```python
from build123d import *

# Parameters (mm, degrees)
F0_W      = 170
F0_H      = 145
F1_DEPTH  = 2
F2_R      = 2.45
F3_DEPTH  = 33
F4_W      = 10
F4_H      = 10
F5_DEPTH  = 20
F8_DEPTH  = 2
F9_W      = 8
F9_H      = 8
F10_DEPTH = 2


with BuildPart() as f1:
    # F0 (on Top) → F1 (new body)
    with BuildSketch(Plane.XY):
        with Locations((85, 72.5)):
            Rectangle(F0_W, F0_H)
    extrude(amount=F1_DEPTH)

    # F2 (on face) → F3 (join)
    with BuildSketch(Plane.XY.offset(2)):
        with Locations((22, 135.5)):
            Circle(F2_R)
        with Locations((22, 14.5)):
            Circle(F2_R)
        with Locations((143, 135.5)):
            Circle(F2_R)
        with Locations((143, 14.5)):
            Circle(F2_R)
    extrude(amount=F3_DEPTH)

    # F4 (on face) → F5 (join)
    with BuildSketch(Plane.XY.offset(2)):
        with Locations((85, 14.5)):
            Rectangle(F4_W, F4_H)
        with Locations((85, 135.5)):
            Rectangle(F4_W, F4_H)
        with Locations((22, 72.5)):
            Rectangle(F4_W, F4_H)
        with Locations((148, 72.5)):
            Rectangle(F4_W, F4_H)
    extrude(amount=F5_DEPTH)

    # F7 (on face) → F8 (join)
    with BuildSketch(Plane.XY.offset(2)):
        Polygon((85, 19.5), (27, 72.5), (27, 67.5), (22, 67.5), (80, 14.5), (80, 19.5), align=None)
        Polygon((143, 72.5), (85, 19.5), (90, 19.5), (90, 14.5), (148, 67.5), (143, 67.5), align=None)
        Polygon((90, 130.5), (85, 130.5), (143, 72.5), (143, 77.5), (148, 77.5), (90, 135.5), align=None)
        Polygon((27, 77.5), (27, 72.5), (85, 130.5), (80, 130.5), (80, 135.5), (22, 77.5), align=None)
    extrude(amount=F8_DEPTH)

    # F9 (on face) → F10 (join)
    with BuildSketch(Plane.XY.offset(2)):
        Polygon((31.1801801802, 68.6801801802), (81, 68.6801801802), (81, 76.6801801802), (31.1801801802, 76.6801801802), (27, 72.5), align=None)
        Polygon((81, 126.5), (81, 76.6801801802), (89, 76.6801801802), (89, 126.5), (85, 130.5), align=None)
        with Locations((85, 72.6801801802)):
            Rectangle(F9_W, F9_H)
        Polygon((143, 72.5), (138.8198198198, 68.6801801802), (139.1801801802, 68.6801801802), align=None)
        Polygon((89, 76.6801801802), (89, 68.6801801802), (138.8198198198, 68.6801801802), (143, 72.5), (138.8198198198, 76.6801801802), align=None)
        Polygon((81, 68.6801801802), (81, 23.1551724138), (85, 19.5), (89, 23.1551724138), (89, 68.6801801802), align=None)
    extrude(amount=F10_DEPTH)


solid = f1.part
```
CAD build for the part. Positions are in the model's coordinates, mm. A direction names the side the tool comes from. Give positions to 0.01 mm unless a question says otherwise; leave off trailing zeros. Loops run counter-clockwise (first coordinate to the right, second up) from the corner with the lowest first, then second, coordinate; pieces in that order, holes last. Notation, with made-up numbers: (-31, 20.5) - (27, 20.5) arc R19 cw to (27, 41.5) - close; hole circle Ø3 at (36, 74.5). An arc over 180 degrees is marked (long way). Put each result on its own line as item: value.
Q1. Tool access for faces 1 (the face through (145.263, 13.562, 18.269)), 2 (the face through (27, 72, 13)), 3 (the face through (17, 72, 12)), 4 (the face through (143, 15, 35)): list every direction of +Z, -Z, +X, -X, +Y, -Y with a clear straight run to the whole face (end or side of a thin tool).
Filled in:
face 1: +Z
face 2: +Z, +Y, -Y
face 3: +Z, -X, +Y, -Y
face 4: +Z, +X, -X, +Y, -Y
Q2. Slice it at A-A (y = 86.5). Give the cut face in (x, z).
Filled in:
outline: (0, 0) - (170, 0) - (170, 2) - (139, 2) - (139, 4) - (129, 4) - (129, 2) - (89, 2) - (89, 4) - (81, 4) - (81, 2) - (41, 2) - (41, 4) - (31, 4) - (31, 2) - (0, 2) - close
Q3. Probe line 1 along Z through (x, y) = (151, 130); line 2 along Y through (x, z) = (101, 3.5); line 3 along Z through (x, y) = (35, 70). List the from-to ranges inside material, lowest first.
Filled in:
line 1: z = 0 to 2
line 2: y = 24.55 to 34.12, 68.68 to 76.68, 114.5 to 124.5
line 3: z = 0 to 4
Q4. Mould opens along Y. For faces 5 (the face through (85, 9.5, 12)), 6 (the face through (20.056, 13.009, 18.269)), 7 (the face through (84, 74, 0)), 8 (the face through (143, 72, 13)) say: pulls with the +Y half, pulls with the -Y half, needs draft (parallel to the pull), parting line crosses it, or undercut.
Filled in:
face 5: pulls with the -Y half
face 6: undercut
face 7: needs draft
face 8: undercut
Q5. Flat gauge pins, fed straight in: pin 1 (10 mm diameter, centred on y = 31, z = 13, fed in from -X); pin 2 (11 mm diameter, centred on x = 84.5, z = 8.5, fed in from +Y); pin 3 (3 mm diameter, centred on y = 136, z = 13.5, fed in from -X); pin 4 (5 mm diameter, centred on x = 146.5, z = 14.5, fed in from -Y). Where does each tip first touch, or does it go through?
Filled in:
pin 1: passes through
pin 2: stops at y = 140.5
pin 3: stops at x = 19.55
pin 4: stops at y = 12.26
Q6. Slice it at C-C (z = 25.5). Give the cut face in (x, y), plus the area to 3 significant figures.
Filled in:
outline: circle Ø4.9 at (22, 14.5); circle Ø4.9 at (22, 135.5); circle Ø4.9 at (143, 14.5); circle Ø4.9 at (143, 135.5)
area: 75.4 mm²
Q7. Slice it at B-B (z = 16). Give the cut face in (x, y), plus the area to 3 significant figures.
Filled in:
outline: (17, 67.5) - (27, 67.5) - (27, 77.5) - (17, 77.5) - close; circle Ø4.9 at (22, 14.5); circle Ø4.9 at (22, 135.5); (80, 9.5) - (90, 9.5) - (90, 19.5) - (80, 19.5) - close; (80, 130.5) - (90, 130.5) - (90, 140.5) - (80, 140.5) - close; circle Ø4.9 at (143, 14.5); circle Ø4.9 at (143, 135.5); (143, 67.5) - (153, 67.5) - (153, 77.5) - (143, 77.5) - close
area: 475 mm²
Q8. Slice it at D-D (x = 71). Give the cut face in (y, z), plus the area to 3 significant figures.
Filled in:
outline: (0, 0) - (145, 0) - (145, 2) - (126.5, 2) - (126.5, 4) - (116.5, 4) - (116.5, 2) - (76.68, 2) - (76.68, 4) - (68.68, 4) - (68.68, 2) - (32.29, 2) - (32.29, 4) - (22.72, 4) - (22.72, 2) - (0, 2) - close
area: 345 mm²
